The listing builds one solid part. Answer for the finished solid, in the listing's coordinates (mm). A direction names the side the tool comes from. Round coordinates to 2 decimals unless told otherwise and drop trailing zeros. Loops run counter-clockwise (first coordinate to the right, second up) from the corner with the lowest first, then second, coordinate; pieces in that order, holes last. Notation, with made-up numbers: M 2.5,7 L 33.5,7 A29 cw 33.5,43 Z; hole C 55.5,43.25 d9. An arc over 180 degrees is marked long. Put each result on its own line as item: value. Start each with the question number.
(1) Flat-ended cylindrical pins translate along their axes: P1, Ø4, axis at x = -7, y = 4.5, coming from the +Z side; P2, Ø13, axis at x = 0, z = -3.5, coming from the +Y side; P3, Ø4.5, axis at y = 2, z = 4, coming from the +X side; P4, Ø2, axis at y = 3, z = 4, coming from the +X side. Find the tip coordinate at first contact, or state that the pin passes through.
(2) Section D-D, the plane y = 2 is taken. Determine the outline of the cut face in (x, z).
(3) Straight lines are drawn through the part: line 1 (X direction, y = 1.2, z = 0); line 2 (Z direction, x = 13.25, y = 7.25); line 3 (Y direction, x = -1.25, z = -8.25). For each, find the intervals that lie inside material, in ascending order.
(4) Section A-A, the plane z = -4.5 is taken. Determine the outline of the cut face in (x, y), then the cut area to 3 significant figures.
(5) Section B-B, the plane y = 7.5 is taken. Determine the outline of the cut face in (x, z).
(6) Determine the mould class of faces 1 (the face through (11.628, 2, 5)), 2 (the face through (13.66, 5.79, -2.38)), 3 (the face through (10, 3, -14)) for opening direction Z: released by +Z, released by -Z, zero draft, split by the parting line, or undercut.
(7) Section C-C, the plane x = 2.5 is taken. Determine the outline of the cut face in (y, z), then the cut area to 3 significant figures.
(8) Which of the six approach directions +Z, -Z, +X, -X, +Y, -Y give full straight-line access (tool end or side, diameter ignored) to faces 4 (the face through (11.628, 8, -6)), 5 (the face through (14, 11, -6))?
```python
from build123d import *

# Parameters (mm, degrees)
SKETCH1_R           = 6.25
BOSS_EXTRUDE1_DEPTH = 4
SKETCH2_W           = 4.12162106
SKETCH2_H           = 16.002035265
BOSS_EXTRUDE2_DEPTH = 7
SKETCH3_R           = 1.75
CUT_EXTRUDE1_DEPTH  = 32.205988509
FILLET2_R           = 1


with BuildPart() as part:
    # Sketch1 → Boss-Extrude1 (new body)
    with BuildSketch(Plane(origin=(0, 0, 0), x_dir=(1, 0, 0), z_dir=(0, 1, 0))):
        with BuildLine():
            Line((0, 14), (15.749998278, 14))
            Line((15.749998278, 14), (15.749998278, -2.002035265))
            Line((15.749998278, -2.002035265), (11.628377218, -2.002035265))
            Line((11.628377218, -2.002035265), (11.628377218, -7.79620698))
            ThreePointArc((11.628377218, -7.79620698), (-12.352062535, -6.589882483), (0, 14))
        make_face()
        with Locations(Location((0, 0, 0), (0, 0, 270))):
            Circle(SKETCH1_R, mode=Mode.SUBTRACT)
    extrude(amount=BOSS_EXTRUDE1_DEPTH)

    # Sketch2 → Boss-Extrude2 (add)
    with BuildSketch(Plane(origin=(0, 4, 0), x_dir=(1, 0, 0), z_dir=(0, 1, 0))):
        with Locations((13.689187748, 5.998982368)):
            Rectangle(SKETCH2_W, SKETCH2_H)
    extrude(amount=BOSS_EXTRUDE2_DEPTH)

    # Sketch3 → Cut-Extrude1 (cut, through all)
    with BuildSketch(Plane.ZY.offset(-11.628377218)):
        with Locations((-1.998982368, 7.5)):
            Circle(SKETCH3_R)
        with Locations((-9.998982368, 7.5)):
            Circle(SKETCH3_R)
    extrude(amount=-CUT_EXTRUDE1_DEPTH, mode=Mode.SUBTRACT)

    # Fillet2
    fillet2_edges = [part.edges().sort_by_distance(p)[0] for p in [
        (11.628377218, 4, -5.998982368),
    ]]
    fillet(fillet2_edges, radius=FILLET2_R)


solid = part.part
```
Recorded:
1. P1: stops at z = 13.05
1. P2: stops at y = 4
1. P3: stops at x = 15.75
1. P4: stops at x = 11.63
2. outline: M 0,-14 L 15.75,-14 L 15.75,2 L 11.63,2 L 11.63,7.8 A14 ccw long Z; hole C 0,0 d12.5
3. line 1: x = -14 to -6.25, 6.25 to 15.75
3. line 2: z = -14 to -11.73, -8.27 to -3.73, -0.27 to 2
3. line 3: y = 0 to 4
4. outline: M -13.26,0 L -4.34,0 L -4.34,4 L -13.26,4 Z; M 4.34,0 L 15.75,0 L 15.75,11 L 11.63,11 L 11.63,5 A1 cw 10.63,4 L 4.34,4 Z
4. area: 110 mm²
5. outline: M 11.63,-14 L 15.75,-14 L 15.75,-11.75 L 11.63,-11.75 Z; M 11.63,-8.25 L 15.75,-8.25 L 15.75,-3.75 L 11.63,-3.75 Z; M 11.63,-0.25 L 15.75,-0.25 L 15.75,2 L 11.63,2 Z
6. face 1: zero draft
6. face 2: undercut
6. face 3: released by -Z
7. outline: M 0,-14 L 4,-14 L 4,-5.73 L 0,-5.73 Z; M 0,5.73 L 4,5.73 L 4,13.77 L 0,13.77 Z
7. area: 65.3 mm²
8. face 4: +Z, -Z, -X, +Y
8. face 5: +Z, -Z, +X, -X, +Y
